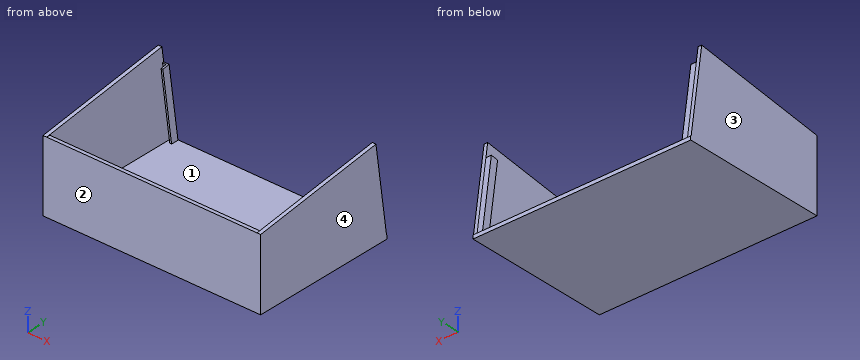
from build123d import *

# Parameters (mm, degrees)
F0_W      = 120
F0_H      = 80
F1_DEPTH  = 2
F3_DEPTH  = 2
F5_W      = 116
F5_H      = 37.1859224175
F6_DEPTH  = 2
F8_DEPTH  = 3
F9_W      = 1.9952932298
F9_H      = 3.2731545162
F10_REACH = 45.8542642129


with BuildPart() as f1:
    # F0 (on Top) → F1 (new body)
    with BuildSketch(Plane.XY):
        with Locations((0, 16.5011590771)):
            Rectangle(F0_W, F0_H)
    extrude(amount=F1_DEPTH)

    # F2 (on face) → F3 (join)
    with BuildSketch(Plane.YZ.offset(60)):
        Polygon((-23.4988409229, 2), (56.2183740699, 2), (49.5011590771, 49.5075751779), (-23.4988409229, 39.1859224175), align=None)
    extrude(amount=-F3_DEPTH)

    # F4: F1 across plane


with BuildPart() as f1_1:
    add(f1.part)
    add(f1.part.mirror(Plane.YZ))

    # F5 (on face) → F6 (join)
    with BuildSketch(Plane.XZ.offset(23.4988409229)):
        with Locations((0, 20.5929612087)):
            Rectangle(F5_W, F5_H)
    extrude(amount=-F6_DEPTH)

    # F7 (on face) → F8 (join)
    with BuildSketch(Plane.YZ.offset(-58)):
        Polygon((52.1785882537, 2), (56.2183740699, 2), (50.6183740699, 41.6060601424), (46.6577680557, 41.0460601424), align=None)
    extrude(amount=F8_DEPTH)

    f10_end = Plane(origin=(0.0757710305, 17.4568088596, 2), x_dir=(1, 0, 0), z_dir=(0, 0, 1))
    # F9 (on face) → F10 (cut, up to a plane its end follows)
    with BuildSketch(Plane(origin=(0, -4.7753622892, 33.7738010765), x_dir=(1, 0, 0), z_dir=(0, -0.14, 0.9901515036))):
        with Locations((-57.0023533851, 53.5812848711)):
            Rectangle(F9_W, F9_H)
    f10_long = extrude(amount=-F10_REACH, mode=Mode.PRIVATE)
    add(split(f10_long, bisect_by=f10_end, keep=Keep.TOP, mode=Mode.PRIVATE), mode=Mode.SUBTRACT)

    # F11: F1 across plane


with BuildPart() as f1_2:
    add(f1_1.part)
    add(f1_1.part.mirror(Plane.YZ))


solid = f1_2.part
Work out the finished part from the listing and answer in its coordinate system (mm). Face numbers are marked on the shaded views. Give positions to 0.01 mm unless a question says otherwise; leave off trailing zeros. Loops run counter-clockwise (first coordinate to the right, second up) from the corner with the lowest first, then second, coordinate; pieces in that order, holes last. Notation, with made-up numbers: (33, -1.5) -> (49, -1.5) arc R25 cw to (49, 37.5) -> close; hole circle Ø1 at (-15, 69.5). An arc over 180 degrees is marked (long way). Use a Markdown table: item, result. Add a question column.
1. Section B-B on y = 26 is taken. Determine the outline of the cut face in (x, z).
2. Flat-ended cylindrical pins translate along their axes: pin 1 Ø5 at (x, z) = (3.5, 18) entering from +Y; pin 2 Ø1 at (x, y) = (10, -3.5) entering from +Z; pin 3 Ø1 at (x, y) = (-19.5, -22) entering from +Z. Find the tip coordinate at first contact, or state that the pin passes through.
3. Section C-C on x = -37 is taken. Determine the outline of the cut face in (y, z), and give its area (3 significant figures).
4. Section D-D on z = 17.5 is taken. Determine the outline of the cut face in (x, y).
5. Find the intervals of material crossed by probe 1 along X at (y, z) = (41.5, 6); probe 2 along Z at (x, y) = (9.5, 14); probe 3 along Y at (x, z) = (2.5, 24.5), in increasing order.
6. Determine the mould class of the marked faces 1, 2, 3 and 4 for opening direction X: released by +X, released by -X, zero draft, split by the parting line, or undercut.
7. Section A-A on z = 43 is taken. Determine the outline of the cut face in (x, y).
Results below:
| question | item | result |
|---|---|---|
| 1 | outline | (-60, 0) -> (60, 0) -> (60, 46.18) -> (58, 46.18) -> (58, 2) -> (-58, 2) -> (-58, 46.18) -> (-60, 46.18) -> close |
| 2 | pin 1 | stops at y = -21.5 |
| 2 | pin 2 | stops at z = 2 |
| 2 | pin 3 | stops at z = 39.19 |
| 3 | outline | (-23.5, 0) -> (56.5, 0) -> (56.5, 2) -> (-21.5, 2) -> (-21.5, 39.19) -> (-23.5, 39.19) -> close |
| 3 | area | 234 mm^2 |
| 4 | outline | (-60, -23.5) -> (60, -23.5) -> (60, 54.03) -> (55, 54.03) -> (55, 49.99) -> (56, 49.99) -> (56, 53.29) -> (58, 53.29) -> (58, -21.5) -> (-58, -21.5) -> (-58, 53.29) -> (-56, 53.29) -> (-56, 49.99) -> (-55, 49.99) -> (-55, 54.03) -> (-60, 54.03) -> close |
| 5 | probe 1 | x = -60 to -58, 58 to 60 |
| 5 | probe 2 | z = 0 to 2 |
| 5 | probe 3 | y = -23.5 to -21.5 |
| 6 | face 1 | undercut |
| 6 | face 2 | zero draft |
| 6 | face 3 | released by -X |
| 6 | face 4 | released by +X |
| 7 | outline | (-60, 3.48) -> (-58, 3.48) -> (-58, 50.42) -> (-60, 50.42) -> close; (58, 3.48) -> (60, 3.48) -> (60, 50.42) -> (58, 50.42) -> close |
